```python
from build123d import *

# Parameters (mm, degrees)
SKETCH1_W           = 28
SKETCH1_H           = 25.1
BOSS_EXTRUDE1_DEPTH = 1.65
SKETCH2_W           = 11.2
SKETCH2_H           = 15
BOSS_EXTRUDE2_DEPTH = 6.2
BOSS_EXTRUDE3_DEPTH = 1
SKETCH4_W           = 6.55
SKETCH4_H           = 11.95
BOSS_EXTRUDE4_DEPTH = 4.5
SKETCH5_R           = 2.525
BOSS_EXTRUDE5_DEPTH = 2
SKETCH6_R           = 0.9
CUT_EXTRUDE1_DEPTH  = 22.074273416


with BuildPart() as part:
    # Sketch1 → Boss-Extrude1 (new body)
    with BuildSketch(Plane(origin=(0, 0, 0), x_dir=(1, 0, 0), z_dir=(0, 1, 0))):
        Rectangle(SKETCH1_W, SKETCH1_H)
    extrude(amount=BOSS_EXTRUDE1_DEPTH)

    # Sketch2 → Boss-Extrude2 (add)
    with BuildSketch(Plane(origin=(0, 1.65, 0), x_dir=(1, 0, 0), z_dir=(0, 1, 0))):
        with Locations((8.4, 0)):
            Rectangle(SKETCH2_W, SKETCH2_H)
    extrude(amount=BOSS_EXTRUDE2_DEPTH)

    # Sketch3 → Boss-Extrude3 (add)
    with BuildSketch(Plane(origin=(14, 0, 0), x_dir=(0, 0, -1), z_dir=(1, 0, 0))):
        Polygon((-7.5, 4.3), (-7.5, 7.85), (7.5, 7.85), (7.5, 4.3), (5.5, 2.3), (-5.5, 2.3), align=None)
    extrude(amount=BOSS_EXTRUDE3_DEPTH)

    # Sketch4 → Boss-Extrude4 (add)
    with BuildSketch(Plane.XZ):
        with Locations((-5.525, 4.075)):
            Rectangle(SKETCH4_W, SKETCH4_H)
    extrude(amount=BOSS_EXTRUDE4_DEPTH)

    # Sketch5 → Boss-Extrude5 (add)
    with BuildSketch(Plane.XY.offset(10.05)):
        with Locations((-5.525, -2.25)):
            Circle(SKETCH5_R)
    extrude(amount=BOSS_EXTRUDE5_DEPTH)

    # Sketch6 → Cut-Extrude1 (cut, through all)
    with BuildSketch(Plane(origin=(0, 0, 0), x_dir=(-1, 0, 0), z_dir=(0, -1, 0))):
        with Locations(Location((11.95, -10.5, 0), (0, 0, 90))):
            Circle(SKETCH6_R)
        with Locations(Location((11.95, 10.5, 0), (0, 0, 90))):
            Circle(SKETCH6_R)
        with Locations(Location((-0.5, 10.5, 0), (0, 0, 90))):
            Circle(SKETCH6_R)
        with Locations(Location((-0.5, -10.5, 0), (0, 0, 90))):
            Circle(SKETCH6_R)
    extrude(amount=-CUT_EXTRUDE1_DEPTH, mode=Mode.SUBTRACT)


solid = part.part
```
Verification items for the finished model (mm, model axes). A direction names the side the tool comes from. Round coordinates to 2 decimals unless told otherwise and drop trailing zeros. Write each loop counter-clockwise with the first axis right and the second up, starting at its lowest first coordinate (ties: lowest second). Pieces come first, ordered by that corner, then holes. Notation, with made-up numbers: (74.5, -31.5) -> (99.5, -31.5) arc R23 cw to (99.5, -13.5) -> close; hole circle Ø4 at (59, 36). An arc over 180 degrees is marked (long way). Write each question's results on one line, items separated by ' | '. Start each with the question number.
1. Set-up check for faces 1 (the flat face through (-2.25, -2, 4)), 2 (the flat face through (14.5, 3.3, 6.5)), 3 (the flat face through (9, 5, -7.5)), 4 (the flat face through (-6, -2, -1.9)): record each of +Z, -Z, +X, -X, +Y, -Y from which the full face is reachable in a straight line by a thin tool's end or side.
2. Cross-section at C-C (y = -2.25). Enter the section's corners in (x, z), then the cut area to 3 significant figures.
3. Cross-section at B-B (x = 0.5). Enter the section's corners in (y, z).
4. Material ranges on probe 1 along X at (y, z) = (0.95, 10.5); probe 2 along Z at (x, y) = (-12.75, 0.5); probe 3 along Z at (x, y) = (10.75, 5), recorded low to high. Write a range as from..to.
5. Draft check along X on faces 5 (the flat face through (15, 5, 0)), 6 (the flat face through (-14, 1, 0)), 7 (the cylindrical face through (0.77, 0.81, -11.36)), 8 (the flat face through (-3, 1.65, 0)). Enter one of: +X half, -X half, draft (parallel to the pull), parting line (faces both ways), or undercut.
6. Cross-section at A-A (z = -10.5). Enter the section's corners in (x, y).
7. Depth check by flat-ended pin: P1, Ø12, axis at x = 4.5, z = -3, coming from the -Y side; P2, Ø2, axis at x = -7, z = 5.5, coming from the -Y side; P3, Ø1.5, axis at x = 10, y = 6.5, coming from the -Z side. Enter the tip coordinate at first touch or a pass-through.
8. Cross-section at D-D (x = 11). Enter the section's corners in (y, z), then the cut area to 3 significant figures.
Solutions:
1) face 1: +Z, -Z, +X, -Y | face 2: +Z, +X, -Y | face 3: -Z, +X, -X, +Y | face 4: -Z, +X, -X, -Y
2) outline: (-8.8, -1.9) -> (-2.25, -1.9) -> (-2.25, 10.05) -> (-3, 10.05) -> (-3, 12.05) -> (-8.05, 12.05) -> (-8.05, 10.05) -> (-8.8, 10.05) -> close | area: 88.4 mm2
3) outline: (0, -12.55) -> (1.65, -12.55) -> (1.65, -11.4) -> (0, -11.4) -> close; (0, -9.6) -> (1.65, -9.6) -> (1.65, 9.6) -> (0, 9.6) -> close; (0, 11.4) -> (1.65, 11.4) -> (1.65, 12.55) -> (0, 12.55) -> close
4) probe 1: x = -14..-12.85, -11.05..-0.4, 1.4..14 | probe 2: z = -12.55..-10.91, -10.09..10.09, 10.91..12.55 | probe 3: z = -7.5..7.5
5) face 5: +X half | face 6: -X half | face 7: undercut | face 8: draft
6) outline: (-14, 0) -> (-12.85, 0) -> (-12.85, 1.65) -> (-14, 1.65) -> close; (-11.05, 0) -> (-0.4, 0) -> (-0.4, 1.65) -> (-11.05, 1.65) -> close; (1.4, 0) -> (14, 0) -> (14, 1.65) -> (1.4, 1.65) -> close
7) P1: stops at y = 0 | P2: stops at y = -4.5 | P3: stops at z = -7.5
8) outline: (0, -12.55) -> (1.65, -12.55) -> (1.65, -7.5) -> (7.85, -7.5) -> (7.85, 7.5) -> (1.65, 7.5) -> (1.65, 12.55) -> (0, 12.55) -> close | area: 134 mm2
